For this review, take the finished solid that the model builds, in its own axes (mm). A direction names the side the tool comes from. Give positions to 0.01 mm unless a question says otherwise; leave off trailing zeros. Write each loop counter-clockwise with the first axis right and the second up, starting at its lowest first coordinate (ties: lowest second). Pieces come first, ordered by that corner, then holes. Notation, with made-up numbers: (15, 53.5) -> (29, 53.5) arc R20 cw to (29, 82.5) -> close; hole circle Ø8 at (-16.75, 75). An arc over 180 degrees is marked (long way). Return JSON: item names as keys, results as strings.
from build123d import *

# Parameters (mm, degrees)
BOSS_EXTRUDE4_DEPTH   = 1
BOSS_EXTRUDE5_DEPTH   = 4
CUT_EXTRUDE3_DEPTH    = 6
LPATTERN1_COUNT       = 11
LPATTERN1_PITCH       = 60
MIRROR1_COPY_1_DEPTH  = 6
MIRROR1_COPY_2_DEPTH  = 6
MIRROR1_COPY_3_DEPTH  = 6
MIRROR1_COPY_4_DEPTH  = 6
MIRROR1_COPY_5_DEPTH  = 6
MIRROR1_COPY_6_DEPTH  = 6
MIRROR1_COPY_7_DEPTH  = 6
MIRROR1_COPY_8_DEPTH  = 6
MIRROR1_COPY_9_DEPTH  = 6
MIRROR1_COPY_10_DEPTH = 6


with BuildPart() as part:
    # Sketch3 → Boss-Extrude4 (new body)
    with BuildSketch(Plane.XY):
        with BuildLine():
            Line((-350, 18), (350, 18))
            ThreePointArc((350, 18), (368, 0), (350, -18))
            Line((350, -18), (-350, -18))
            ThreePointArc((-350, -18), (-368, 0), (-350, 18))
        make_face()
    extrude(amount=BOSS_EXTRUDE4_DEPTH)

    # Sketch4 → Boss-Extrude5 (add)
    with BuildSketch(Plane.XY.offset(1)):
        with BuildLine():
            Line((-350, 15), (350, 15))
            ThreePointArc((350, 15), (365, 0), (350, -15))
            Line((350, -15), (-350, -15))
            ThreePointArc((-350, -15), (-365, 0), (-350, 15))
        make_face()
    extrude(amount=BOSS_EXTRUDE5_DEPTH)

    # Sketch5 → Cut-Extrude3 (cut, through all)
    with BuildSketch(Plane.XY.offset(5)):
        with BuildLine():
            Line((-317.5, 11), (-282.5, 11))
            ThreePointArc((-282.5, 11), (-279.5, 8), (-282.5, 5))
            Line((-282.5, 5), (-317.5, 5))
            ThreePointArc((-317.5, 5), (-320.5, 8), (-317.5, 11))
        make_face()
    cut_extrude3 = extrude(amount=-CUT_EXTRUDE3_DEPTH, mode=Mode.SUBTRACT)

    # LPattern1: Cut-Extrude3 ×11
    with Locations(*[(i * LPATTERN1_PITCH, 0, 0) for i in range(1, LPATTERN1_COUNT)]):
        add(cut_extrude3, mode=Mode.SUBTRACT)

    # Mirror1: Cut-Extrude3 across plane
    add(cut_extrude3.mirror(Plane.ZX), mode=Mode.SUBTRACT)

    # Mirror1 copy 1 sketch → Mirror1 copy 1 (cut, through all)
    with BuildSketch(Plane(origin=(60, 0, 5), x_dir=(1, 0, 0), z_dir=(0, 0, 1))):
        with BuildLine():
            Line((-317.5, -11), (-282.5, -11))
            ThreePointArc((-282.5, -11), (-279.5, -8), (-282.5, -5))
            Line((-282.5, -5), (-317.5, -5))
            ThreePointArc((-317.5, -5), (-320.5, -8), (-317.5, -11))
        make_face()
    extrude(amount=-MIRROR1_COPY_1_DEPTH, mode=Mode.SUBTRACT)

    # Mirror1 copy 2 sketch → Mirror1 copy 2 (cut, through all)
    with BuildSketch(Plane(origin=(120, 0, 5), x_dir=(1, 0, 0), z_dir=(0, 0, 1))):
        with BuildLine():
            Line((-317.5, -11), (-282.5, -11))
            ThreePointArc((-282.5, -11), (-279.5, -8), (-282.5, -5))
            Line((-282.5, -5), (-317.5, -5))
            ThreePointArc((-317.5, -5), (-320.5, -8), (-317.5, -11))
        make_face()
    extrude(amount=-MIRROR1_COPY_2_DEPTH, mode=Mode.SUBTRACT)

    # Mirror1 copy 3 sketch → Mirror1 copy 3 (cut, through all)
    with BuildSketch(Plane(origin=(180, 0, 5), x_dir=(1, 0, 0), z_dir=(0, 0, 1))):
        with BuildLine():
            Line((-317.5, -11), (-282.5, -11))
            ThreePointArc((-282.5, -11), (-279.5, -8), (-282.5, -5))
            Line((-282.5, -5), (-317.5, -5))
            ThreePointArc((-317.5, -5), (-320.5, -8), (-317.5, -11))
        make_face()
    extrude(amount=-MIRROR1_COPY_3_DEPTH, mode=Mode.SUBTRACT)

    # Mirror1 copy 4 sketch → Mirror1 copy 4 (cut, through all)
    with BuildSketch(Plane(origin=(240, 0, 5), x_dir=(1, 0, 0), z_dir=(0, 0, 1))):
        with BuildLine():
            Line((-317.5, -11), (-282.5, -11))
            ThreePointArc((-282.5, -11), (-279.5, -8), (-282.5, -5))
            Line((-282.5, -5), (-317.5, -5))
            ThreePointArc((-317.5, -5), (-320.5, -8), (-317.5, -11))
        make_face()
    extrude(amount=-MIRROR1_COPY_4_DEPTH, mode=Mode.SUBTRACT)

    # Mirror1 copy 5 sketch → Mirror1 copy 5 (cut, through all)
    with BuildSketch(Plane(origin=(300, 0, 5), x_dir=(1, 0, 0), z_dir=(0, 0, 1))):
        with BuildLine():
            Line((-317.5, -11), (-282.5, -11))
            ThreePointArc((-282.5, -11), (-279.5, -8), (-282.5, -5))
            Line((-282.5, -5), (-317.5, -5))
            ThreePointArc((-317.5, -5), (-320.5, -8), (-317.5, -11))
        make_face()
    extrude(amount=-MIRROR1_COPY_5_DEPTH, mode=Mode.SUBTRACT)

    # Mirror1 copy 6 sketch → Mirror1 copy 6 (cut, through all)
    with BuildSketch(Plane(origin=(360, 0, 5), x_dir=(1, 0, 0), z_dir=(0, 0, 1))):
        with BuildLine():
            Line((-317.5, -11), (-282.5, -11))
            ThreePointArc((-282.5, -11), (-279.5, -8), (-282.5, -5))
            Line((-282.5, -5), (-317.5, -5))
            ThreePointArc((-317.5, -5), (-320.5, -8), (-317.5, -11))
        make_face()
    extrude(amount=-MIRROR1_COPY_6_DEPTH, mode=Mode.SUBTRACT)

    # Mirror1 copy 7 sketch → Mirror1 copy 7 (cut, through all)
    with BuildSketch(Plane(origin=(420, 0, 5), x_dir=(1, 0, 0), z_dir=(0, 0, 1))):
        with BuildLine():
            Line((-317.5, -11), (-282.5, -11))
            ThreePointArc((-282.5, -11), (-279.5, -8), (-282.5, -5))
            Line((-282.5, -5), (-317.5, -5))
            ThreePointArc((-317.5, -5), (-320.5, -8), (-317.5, -11))
        make_face()
    extrude(amount=-MIRROR1_COPY_7_DEPTH, mode=Mode.SUBTRACT)

    # Mirror1 copy 8 sketch → Mirror1 copy 8 (cut, through all)
    with BuildSketch(Plane(origin=(480, 0, 5), x_dir=(1, 0, 0), z_dir=(0, 0, 1))):
        with BuildLine():
            Line((-317.5, -11), (-282.5, -11))
            ThreePointArc((-282.5, -11), (-279.5, -8), (-282.5, -5))
            Line((-282.5, -5), (-317.5, -5))
            ThreePointArc((-317.5, -5), (-320.5, -8), (-317.5, -11))
        make_face()
    extrude(amount=-MIRROR1_COPY_8_DEPTH, mode=Mode.SUBTRACT)

    # Mirror1 copy 9 sketch → Mirror1 copy 9 (cut, through all)
    with BuildSketch(Plane(origin=(540, 0, 5), x_dir=(1, 0, 0), z_dir=(0, 0, 1))):
        with BuildLine():
            Line((-317.5, -11), (-282.5, -11))
            ThreePointArc((-282.5, -11), (-279.5, -8), (-282.5, -5))
            Line((-282.5, -5), (-317.5, -5))
            ThreePointArc((-317.5, -5), (-320.5, -8), (-317.5, -11))
        make_face()
    extrude(amount=-MIRROR1_COPY_9_DEPTH, mode=Mode.SUBTRACT)

    # Mirror1 copy 10 sketch → Mirror1 copy 10 (cut, through all)
    with BuildSketch(Plane(origin=(600, 0, 5), x_dir=(1, 0, 0), z_dir=(0, 0, 1))):
        with BuildLine():
            Line((-317.5, -11), (-282.5, -11))
            ThreePointArc((-282.5, -11), (-279.5, -8), (-282.5, -5))
            Line((-282.5, -5), (-317.5, -5))
            ThreePointArc((-317.5, -5), (-320.5, -8), (-317.5, -11))
        make_face()
    extrude(amount=-MIRROR1_COPY_10_DEPTH, mode=Mode.SUBTRACT)


solid = part.part
1. Add section C-C, the plane z = 2.6. Count the separate pieces of the cut face and the enclosed holes in it, plus the area to 3 significant figures.
Results found:
{"separate pieces": "1", "enclosed holes": "22", "area": "16,500 mm²"}
2. Add section A-A, the plane x = -244.5. State the section outline as (y, z) points, plus the area to 3 significant figures.
Results found:
{"outline": "(-18, 0) -> (-11, 0) -> (-11, 5) -> (-15, 5) -> (-15, 1) -> (-18, 1) -> close; (-5, 0) -> (5, 0) -> (5, 5) -> (-5, 5) -> close; (11, 0) -> (18, 0) -> (18, 1) -> (15, 1) -> (15, 5) -> (11, 5) -> close", "area": "96.0 mm²"}
3. For faces 1 (the cylindrical face through (365, 0, 3)), 2 (the cylindrical face through (-365, 0, 3)), 3 (the cylindrical face through (-367.996, -0.396, 0.493)), list the 3-axis set-ups (+Z, -Z, +X, -X, +Y, -Y) from which the entire face can be reached by the end or side of a thin tool; tool diameter is ignored.
Results found:
{"face 1": "+Z, +X", "face 2": "+Z, -X", "face 3": "+Z, -Z, -X"}
4. For pin 1 (2 mm diameter, centred on x = 264.5, y = 13.5, fed in from -Z); pin 2 (1.5 mm diameter, centred on x = -246, z = 3.5, fed in from +Y); pin 3 (1.5 mm diameter, centred on x = -235, z = 2, fed in from -Y), all flat-tipped, find the tip position at first contact; note any pin that passes through.
Results found:
{"pin 1": "stops at z = 0", "pin 2": "stops at y = 15", "pin 3": "stops at y = -15"}
5. To check wall thickness, follow probe 1 along Y at (x, z) = (8, 1.5); probe 2 along Y at (x, z) = (-102, 0.4); probe 3 along Y at (x, z) = (159, 4.8). State the ranges of each line that lie inside material, in increasing order.
Results found:
{"probe 1": "y = -15 to -11, -5 to 5, 11 to 15", "probe 2": "y = -18 to -10.96, -5.04 to 5.04, 10.96 to 18", "probe 3": "y = -15 to 15"}
6. Add section B-B, the plane x = 92.5. State the section outline as (y, z) points.
Results found:
{"outline": "(-18, 0) -> (18, 0) -> (18, 1) -> (15, 1) -> (15, 5) -> (-15, 5) -> (-15, 1) -> (-18, 1) -> close"}
